The listing builds one solid part. Answer for the finished solid, in the listing's coordinates (mm). Coordinates: 2 decimals unless noted, no trailing zeros. Put each result on its own line as item: value.
```python
from build123d import *

# Parameters (mm, degrees)
SKETCH1_W                   = 141.287862113
SKETCH1_H                   = 330.949999988
BOSS_EXTRUDE1_DEPTH         = 19.05
HOLE1_D                     = 3.175
HOLE1_DEPTH                 = 31.75
HOLE1_CSINK_D               = 10.16
HOLE1_CSINK_ANGLE           = 82
HOLE1_TIP                   = 0.953866233
HOLE3_D                     = 3.175
HOLE3_DEPTH                 = 38.1
HOLE3_CSINK_D               = 10.16
HOLE3_CSINK_ANGLE           = 82
HOLE3_TIP                   = 0.953866233
F_1_4_0_25_DIAMETER_HOLE1_D = 6.35
HOLE4_D                     = 3.175
HOLE4_DEPTH                 = 31.75
HOLE4_CSINK_D               = 10.16
HOLE4_CSINK_ANGLE           = 82
HOLE4_TIP                   = 0.953866233
HOLE5_D                     = 3.175
HOLE5_DEPTH                 = 38.1
HOLE5_CSINK_D               = 10.16
HOLE5_CSINK_ANGLE           = 82
HOLE5_TIP                   = 0.953866233


with BuildPart() as part:
    # Sketch1 → Boss-Extrude1 (new body)
    with BuildSketch(Plane.XY):
        with Locations((279.996898238, -72.024999997)):
            Rectangle(SKETCH1_W, SKETCH1_H)
    extrude(amount=BOSS_EXTRUDE1_DEPTH)

    # Hole1
    with Locations(Plane(origin=(196.652967181, -72.024999997, 386.262770337), x_dir=(0, 1, 0), z_dir=(-1, 0, 0))):
        with Locations((174.999999994, 685.961004241), (174.999999994, 549.837259632), (174.999999994, 413.713515022), (81.549999997, 779.649723129), (81.549999997, 652.344645962), (62.499999997, 662.953402392), (62.499999997, 769.040966698), (-62.499999997, 769.040966698), (-62.499999997, 662.953402392), (-81.549999997, 652.344645962), (-81.549999997, 779.649723129), (-174.999999994, 413.713515022), (-174.999999994, 549.837259632), (-174.999999994, 685.961004241), (-82.737499997, 600.384620239), (0, 600.384620239), (82.737499997, 600.384620239), (0, 376.737770337), (-82.737499997, 376.737770337), (82.737499997, 376.737770337)):
            CounterSinkHole(HOLE1_D / 2, HOLE1_CSINK_D / 2, depth=HOLE1_DEPTH, counter_sink_angle=HOLE1_CSINK_ANGLE)
            with Locations((0, 0, -(HOLE1_DEPTH + HOLE1_TIP / 2))):  # 118° drill point
                Cone(0, HOLE1_D / 2, HOLE1_TIP, mode=Mode.SUBTRACT)

    # Hole3
    with Locations(Plane(origin=(-181.039434513, 112.499999997, 386.262770337), x_dir=(0.927183855, 0, -0.374606593), z_dir=(0, 1, 0))):
        with Locations((46.221112845, 113.488854888), (39.39759596, 37.945520226), (412.28786892, 80.423559293), (407.308516105, 25.297013484), (513.561319184, 161.164706775), (597.46020397, 127.267357003), (610.543339245, 159.649253123), (694.322923815, 367.011001477), (526.644454459, 193.546602895), (610.424039029, 400.908351249)):
            CounterSinkHole(HOLE3_D / 2, HOLE3_CSINK_D / 2, depth=HOLE3_DEPTH, counter_sink_angle=HOLE3_CSINK_ANGLE)
            with Locations((0, 0, -(HOLE3_DEPTH + HOLE3_TIP / 2))):  # 118° drill point
                Cone(0, HOLE3_D / 2, HOLE3_TIP, mode=Mode.SUBTRACT)

    # 1/4 (0.25) Diameter Hole1 (through all)
    with Locations(Plane(origin=(0, 0, 0), x_dir=(-1, 0, 0), z_dir=(0, 0, -1))):
        with Locations((-312.540829294, -72.024999997)):
            Hole(F_1_4_0_25_DIAMETER_HOLE1_D / 2)

    # Hole4
    with Locations(Plane(origin=(196.652967181, -72.024999997, 609.909620239), x_dir=(0, 1, 0), z_dir=(-1, 0, 0))):
        with Locations((174.999999994, 685.961004241), (174.999999994, 549.837259632), (174.999999994, 413.713515022), (81.549999997, 779.649723129), (81.549999997, 652.344645962), (62.499999997, 662.953402392), (62.499999997, 769.040966698), (-62.499999997, 769.040966698), (-62.499999997, 662.953402392), (-81.549999997, 652.344645962), (-81.549999997, 779.649723129), (-174.999999994, 413.713515022), (-174.999999994, 549.837259632), (-174.999999994, 685.961004241), (-82.737499997, 600.384620239), (0, 600.384620239), (82.737499997, 600.384620239), (0, 376.737770337), (-82.737499997, 376.737770337), (82.737499997, 376.737770337)):
            CounterSinkHole(HOLE4_D / 2, HOLE4_CSINK_D / 2, depth=HOLE4_DEPTH, counter_sink_angle=HOLE4_CSINK_ANGLE)
            with Locations((0, 0, -(HOLE4_DEPTH + HOLE4_TIP / 2))):  # 118° drill point
                Cone(0, HOLE4_D / 2, HOLE4_TIP, mode=Mode.SUBTRACT)

    # Hole5
    with Locations(Plane(origin=(-181.039434513, 112.499999997, 609.909620239), x_dir=(0.927183855, 0, -0.374606593), z_dir=(0, 1, 0))):
        with Locations((46.221112845, 113.488854888), (39.39759596, 37.945520226), (412.28786892, 80.423559293), (407.308516105, 25.297013484), (513.561319184, 161.164706775), (597.46020397, 127.267357003), (610.543339245, 159.649253123), (694.322923815, 367.011001477), (526.644454459, 193.546602895), (610.424039029, 400.908351249)):
            CounterSinkHole(HOLE5_D / 2, HOLE5_CSINK_D / 2, depth=HOLE5_DEPTH, counter_sink_angle=HOLE5_CSINK_ANGLE)
            with Locations((0, 0, -(HOLE5_DEPTH + HOLE5_TIP / 2))):  # 118° drill point
                Cone(0, HOLE5_D / 2, HOLE5_TIP, mode=Mode.SUBTRACT)


solid = part.part
```
1) Straight lines are drawn through the part: L1, parallel to Y at x = 218, z = 8.75; L2, parallel to Y at x = 310.5, z = 4.5. For each, find the intervals that lie inside material, in ascending order. Write a range as [from, to].
Found:
L1: y = [-237.5, -156.15], [-153.38, -73.41], [-70.64, 9.33], [12.1, 93.45]
L2: y = [-237.5, -74.46], [-69.59, 93.45]
2) This flat-tipped pin is pushed along its axis until it touches: pin 1 (3 mm diameter, centred on x = 325.24, z = 9.53, fed in from +Y). Where does it stop, or does it pass through?
Found:
pin 1: stops at y = 74.35
3) For a pull along X with two mould halves and no side action, classify faces 1 (the face through (350.641, -74, 9)), 2 (the face through (309.37, -71.89, 9.66)), 3 (the face through (279, -70, 0)), 4 (the face through (209.353, -74, 9)) as pulls with the +X half, pulls with the -X half, needs draft (parallel to the pull), parting line crosses it, or undercut.
Found:
face 1: pulls with the +X half
face 2: undercut
face 3: needs draft
face 4: pulls with the -X half
